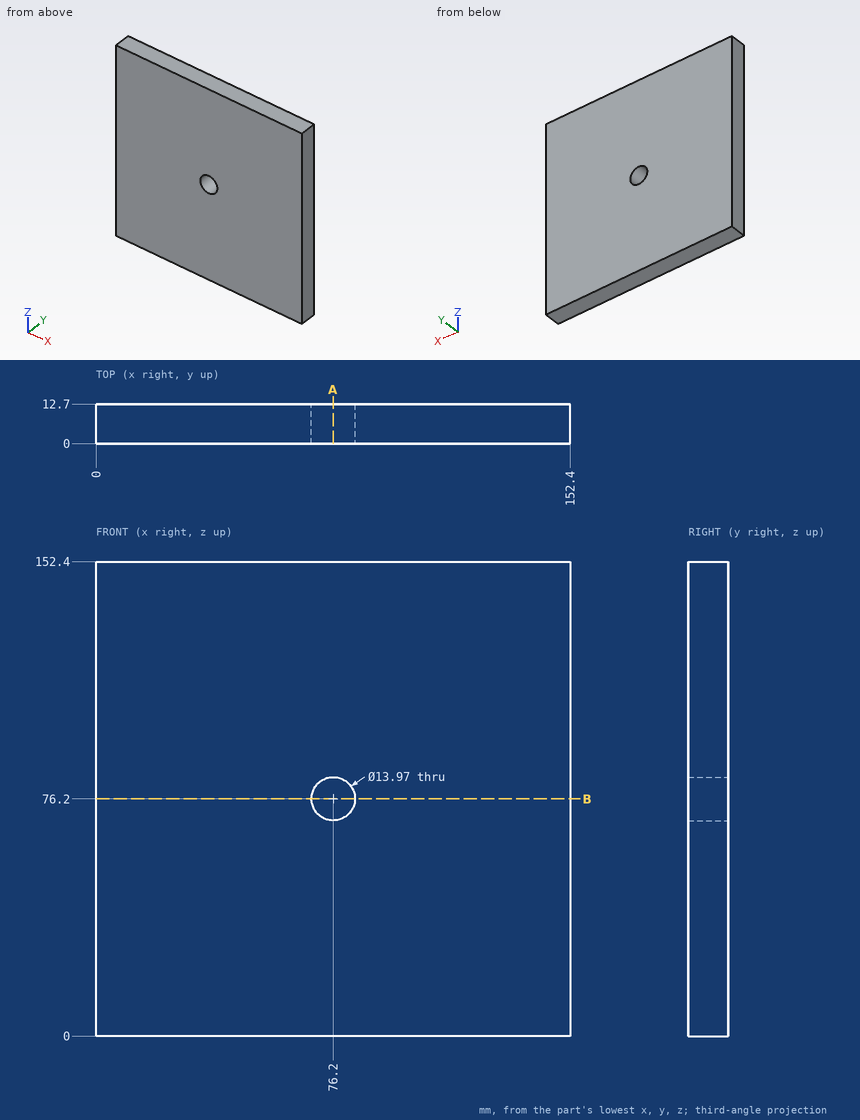
Drawing for the job (mm, zero at the part's lowest x, y, z). Give positions to 0.01 mm unless a question says otherwise; leave off trailing zeros. Order: outer loops, then holes, each group sorted by start corner. A loop starts at its lowest first (then second) coordinate and runs counter-clockwise, first axis right, second up. Notation, with made-up numbers: M 47,42.25 L 90,42.25 A16 cw 90,54.25 Z; hole C 25.25,-1 d9. An arc over 180 degrees is marked long. Use a Markdown table: item, result. Add a question column.
(1) Probe line 1 along Z through (x, y) = (76.2, 5) (3 decimals); line 2 along X through (y, z) = (7.5, 78.5). List the from-to ranges inside material, lowest first. Write a range as [from, to].
(2) Saw through at B-B, the plane z = 76.2. Give the cut face in (x, y) (3 decimals).
(3) Saw through at A-A, the plane x = 76.2. Give the cut face in (y, z) (3 decimals).
Answer key:
| question | item | result |
|---|---|---|
| 1 | line 1 | [0, 69.215], [83.185, 152.4] |
| 1 | line 2 | [0, 69.6], [82.8, 152.4] |
| 2 | outline | M 0,0 L 69.215,0 L 69.215,12.7 L 0,12.7 Z; M 83.185,0 L 152.4,0 L 152.4,12.7 L 83.185,12.7 Z |
| 3 | outline | M 0,0 L 12.7,0 L 12.7,69.215 L 0,69.215 Z; M 0,83.185 L 12.7,83.185 L 12.7,152.4 L 0,152.4 Z |
